```python
from build123d import *

# Parameters (mm, degrees)
PAD_DEPTH    = 15
SKETCH001_W  = 3
SKETCH001_H  = 14
POCKET_DEPTH = 13


with BuildPart() as part:
    # Sketch → Pad (new body)
    with BuildSketch(Plane.XZ):
        with BuildLine():
            ThreePointArc((8.694826, 1.9), (-8.9, 0), (8.694826, -1.9))
            Line((9.994826, -1.9), (8.694826, -1.9))
            Line((9.994826, 1.9), (9.994826, -1.9))
            Line((8.694826, 1.9), (9.994826, 1.9))
        make_face()
    extrude(amount=PAD_DEPTH)

    # Sketch001 (on Face6 of Pad) → Pocket (cut)
    with BuildSketch(Plane.XZ.offset(15)):
        Rectangle(SKETCH001_W, SKETCH001_H)
    extrude(amount=-POCKET_DEPTH, mode=Mode.SUBTRACT)


solid = part.part
```
The listing builds one solid part. Answer for the finished solid, in the listing's coordinates (mm). A direction names the side the tool comes from. Coordinates: 2 decimals unless noted, no trailing zeros. Loops run counter-clockwise (first coordinate to the right, second up) from the corner with the lowest first, then second, coordinate; pieces in that order, holes last. Notation, with made-up numbers: M -3,-27.5 L 55,-27.5 A9 ccw 55,-20.5 Z; hole C 63,87 d6. An arc over 180 degrees is marked long. Answer as a JSON object with one key per item and string values. Group by question number.
Item 1: Section A-A (y = -5.25) is taken. Write down the section's boundary in (x, z), and give its area (3 significant figures).
Item 2: Consider L1, parallel to X at y = -4.5, z = -5.5; L2, parallel to X at y = -7.75, z = 4.75; L3, parallel to Y at x = 1, z = -5.75. Determine where each line is inside the solid, lowest interval first.
Item 3: Which of the six approach directions +Z, -Z, +X, -X, +Y, -Y give full straight-line access (tool end or side, diameter ignored) to faces 5 (the face through (9, -7, -1.9)), 6 (the face through (1.5, -9, 0)), 7 (the face through (-8.893, -7.395, 0.365))?
Item 4: Section B-B (z = 0) is taken. Write down the section's boundary in (x, y), and give its area (3 significant figures).
Item 5: Section D-D (x = -6.5) is taken. Write down the section's boundary in (y, z), and give its area (3 significant figures).
Item 6: Each of these flat-tipped pins is pushed along its axis until it touches: P1, Ø6, axis at x = -6.5, z = 6.5, coming from the -Y side; P2, Ø2, axis at y = -9, z = 2.5, coming from the -X side; P3, Ø1, axis at x = 9.5, y = -8, coming from the +Z side; P4, Ø6, axis at x = -5.5, y = -7, coming from the +Z side. Where does it stop, or does it pass through?
Item 7: Section C-C (x = 0) is taken. Write down the section's boundary in (y, z).
Item 8: Determine the mould class of faces 1 (the face through (0, -9, 7)), 2 (the face through (0, 0, 0)), 3 (the face through (0, -9, -7)), 4 (the face through (9, -7, 1.9)) for opening direction Z: +Z half, -Z half, draft (parallel to the pull), parting line (faces both ways), or undercut.
Solved:
{
 "1": {"outline": "M 8.69,-1.9 L 9.99,-1.9 L 9.99,1.9 L 8.69,1.9 A8.9 ccw long Z; hole M -1.5,-7 L 1.5,-7 L 1.5,7 L -1.5,7 Z", "area": "211 mm2"},
 "2": {"L1": "x = -7 to -1.5, 1.5 to 7", "L2": "x = -7.53 to -1.5, 1.5 to 7.53", "L3": "y = -2 to 0"},
 "3": {"face 5": "-Z, +X, +Y, -Y", "face 6": "-Y", "face 7": "+Y, -Y"},
 "4": {"outline": "M -8.9,-15 L -1.5,-15 L -1.5,-2 L 1.5,-2 L 1.5,-15 L 9.99,-15 L 9.99,0 L -8.9,0 Z", "area": "244 mm2"},
 "5": {"outline": "M -15,-6.08 L 0,-6.08 L 0,6.08 L -15,6.08 Z", "area": "182 mm2"},
 "6": {"P1": "stops at y = -15", "P2": "stops at x = -8.77", "P3": "stops at z = 1.9", "P4": "stops at z = 8.54"},
 "7": {"outline": "M -15,-8.9 L 0,-8.9 L 0,8.9 L -15,8.9 L -15,7 L -2,7 L -2,-7 L -15,-7 Z"},
 "8": {"face 1": "undercut", "face 2": "draft", "face 3": "undercut", "face 4": "+Z half"}
}
